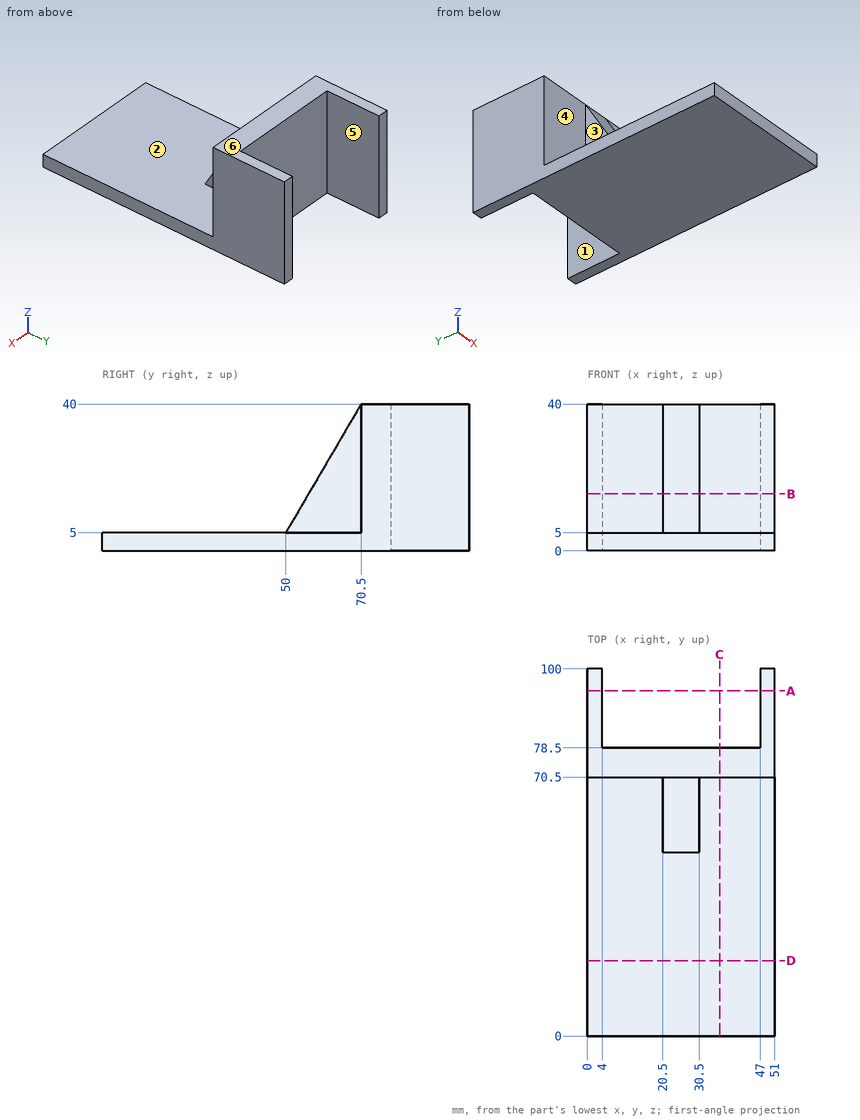
Part print with two shaded views. Sizes in mm from the minimum x, y, z corner. A direction names the side the tool comes from. Give positions to 0.01 mm unless a question says otherwise; leave off trailing zeros. Order: outer loops, then holes, each group sorted by start corner. A loop starts at its lowest first (then second) coordinate and runs counter-clockwise, first axis right, second up.
1) Wall check: probe 1 along X at (y, z) = (82, 14.5); probe 2 along Z at (x, y) = (3.5, 25); probe 3 along Y at (x, z) = (4.5, 22). Give the ranges that are in metal, low to high.
2) Saw through at A-A, the plane y = 94. Write the cut outline in (x, z).
3) Pin check, flat tips, straight feed: pin 1 (23.5 mm diameter, centred on y = 92.5, z = 22, fed in from -X); pin 2 (4 mm diameter, centred on x = 44.5, z = 27, fed in from -Y); pin 3 (6 mm diameter, centred on y = 59, z = 21, fed in from -X); pin 4 (12 mm diameter, centred on x = 19, z = 15, fed in from +Y). Stop position of each tip, or through.
4) Saw through at C-C, the plane x = 36. Write the cut outline in (y, z), then the cut area to 4 significant figures.
5) 3-axis set-ups, long thin cutter, end or side, ignore diameter. For the marked faces 4, 5 and 6: which of +Z, -Z, +X, -X, +Y, -Y reach the whole face in a straight line?
6) Saw through at B-B, the plane z = 15.5. Write the cut outline in (x, y), then the cut area to 4 significant figures.
7) Saw through at D-D, the plane y = 20.5. Write the cut outline in (x, z).
8) Mould opens along X. For the marked faces 1, 2 and 3 say: +X half, -X half, draft (parallel to the pull), parting line (faces both ways), or undercut.
Computed:
1. probe 1: x = 0 to 4, 47 to 51
1. probe 2: z = 0 to 5
1. probe 3: y = 70.5 to 78.5
2. outline: (0, 0) - (4, 0) - (4, 40) - (0, 40) - close; (47, 0) - (51, 0) - (51, 40) - (47, 40) - close
3. pin 1: stops at x = 0
3. pin 2: stops at y = 70.5
3. pin 3: stops at x = 20.5
3. pin 4: stops at y = 78.5
4. outline: (0, 0) - (78.5, 0) - (78.5, 40) - (70.5, 40) - (70.5, 5) - (0, 5) - close
4. area: 672.5 mm2
5. face 4: +Z, -X, -Y
5. face 5: +Z, -Z, +Y
5. face 6: +Z, +X, -X, +Y, -Y
6. outline: (0, 70.5) - (20.5, 70.5) - (20.5, 56.15) - (30.5, 56.15) - (30.5, 70.5) - (51, 70.5) - (51, 100) - (47, 100) - (47, 78.5) - (4, 78.5) - (4, 100) - (0, 100) - close
6. area: 723.5 mm2
7. outline: (0, 0) - (51, 0) - (51, 5) - (0, 5) - close
8. face 1: undercut
8. face 2: draft
8. face 3: -X half
